Verification items for this drawing (mm, ordinates from the low corner). A direction names the side the tool comes from. Coordinates: 2 decimals unless noted, no trailing zeros. Write each loop counter-clockwise with the first axis right and the second up, starting at its lowest first coordinate (ties: lowest second). Pieces come first, ordered by that corner, then holes.
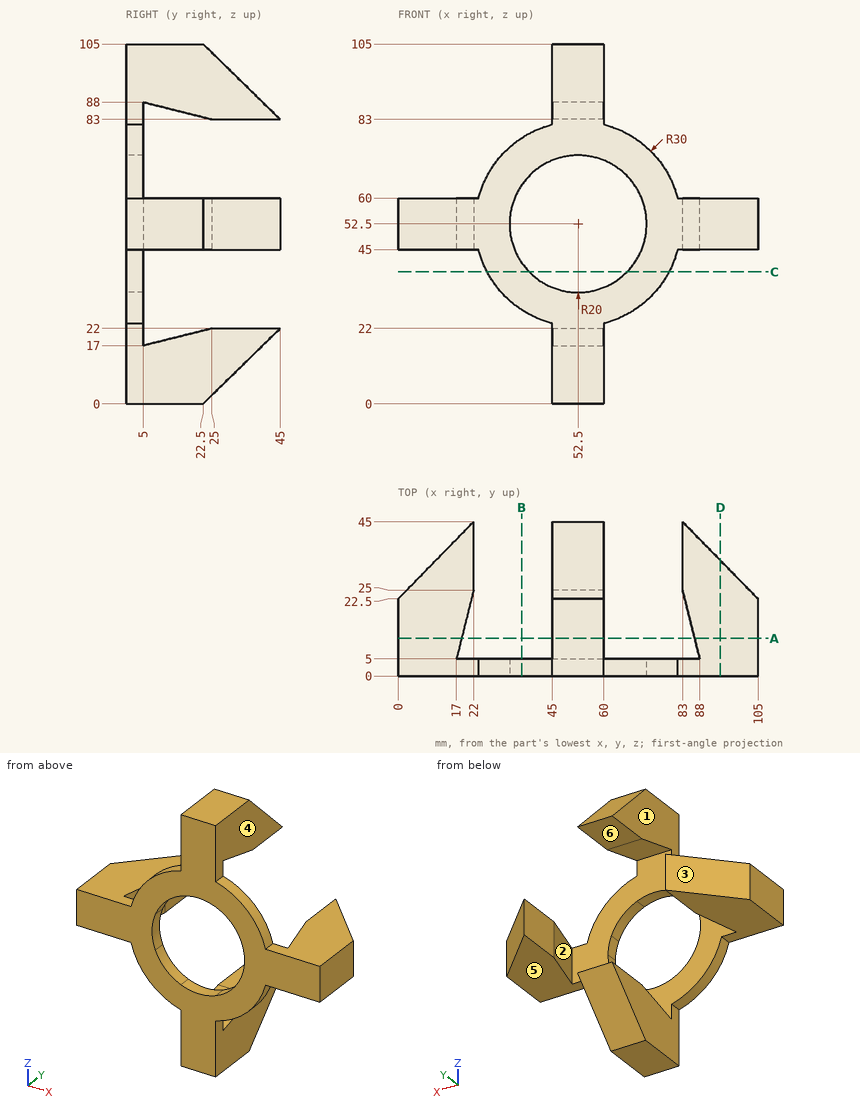
1. Sectioned sample at B-B, the plane x = 36. Record the boundary of the cut face in (y, z), and give its area (3 significant figures).
Computed values:
outline: (0, 27.45) - (5, 27.45) - (5, 41.2) - (0, 41.2) - close; (0, 63.8) - (5, 63.8) - (5, 77.55) - (0, 77.55) - close
area: 138 mm2
2. Draft check along Y on the marked faces 1, 2 and 3. Enter one of: released by +Y, released by -Y, zero draft, split by the parting line, or undercut.
Computed values:
face 1: zero draft
face 2: undercut
face 3: released by +Y
3. Sectioned sample at A-A, the plane y = 11. Record the boundary of the cut face in (x, z), and give its area (3 significant figures).
Computed values:
outline: (0, 45) - (18.5, 45) - (18.5, 60) - (0, 60) - close; (45, 0) - (60, 0) - (60, 18.5) - (45, 18.5) - close; (45, 86.5) - (60, 86.5) - (60, 105) - (45, 105) - close; (86.5, 45) - (105, 45) - (105, 60) - (86.5, 60) - close
area: 1,110 mm2
4. Sectioned sample at C-C, the plane z = 38.5. Record the boundary of the cut face in (x, y).
Computed values:
outline: (25.97, 0) - (38.22, 0) - (38.22, 5) - (25.97, 5) - close; (66.78, 0) - (79.03, 0) - (79.03, 5) - (66.78, 5) - close
5. Thickness scan on line 1 along X through (y, z) = (8, 89.5); line 2 along Y through (x, z) = (40, 26). Record the ranges inside material, lowest first.
Computed values:
line 1: x = 45 to 60
line 2: y = 0 to 5
6. Access from +Z, -Z, +X, -X, +Y, -Y to the whole of each face (thin tool, end or side, straight path). Record for the marked faces 4, 5 and 6.
Computed values:
face 4: +Z, +X, +Y, -Y
face 5: -Z, +X, +Y, -Y
face 6: +X, -X, +Y
7. Sectioned sample at D-D, the plane x = 94. Record the boundary of the cut face in (y, z).
Computed values:
outline: (0, 45) - (33.75, 45) - (33.75, 60) - (0, 60) - close
8. Gauge pin test, flat ends, axial feed: pin 1 Ø8 at (y, z) = (19, 83.5) entering from +X; pin 2 Ø11.5 at (x, y) = (95.5, 33.5) entering from -Z; pin 3 Ø19 at (y, z) = (26, 91) entering from -X; pin 4 Ø12 at (x, z) = (56, 44) entering from +Y. Record the tip position at first contact, or that the pin passes through.
Computed values:
pin 1: stops at x = 60
pin 2: stops at z = 45
pin 3: stops at x = 45
pin 4: passes through
